Geometry check sheet. Reference: the model listing, model coordinates, mm. Face numbers are marked on the shaded views. Coordinates: 2 decimals unless noted, no trailing zeros. Order: outer loops, then holes, each group sorted by start corner. A loop starts at its lowest first (then second) coordinate and runs counter-clockwise, first axis right, second up. Notation, with made-up numbers: (-22.75, -8.5) - (-1.75, -8.5) arc R12 cw to (-1.75, -0.5) - close; hole circle Ø3 at (58, 37.5). An arc over 180 degrees is marked (long way). Use CSV: the item, a comma, the result in double quotes. Start each with the question number.
1) Draft check along X on the marked faces 1, 2, 3 and 4. Enter one of: released by +X, released by -X, zero draft, split by the parting line, or undercut.
2) Sectioned sample at C-C, the plane z = 6.75. Record the cut outline in (x, y).
3) Thickness scan on probe 1 along Y at (x, z) = (0, 8); probe 2 along X at (y, z) = (-10, 1.25); probe 3 along Y at (x, z) = (2.5, 4). Record the ranges inside material, lowest first. Write a range as [from, to].
4) Sectioned sample at A-A, the plane x = 0. Record the cut outline in (y, z).
5) Sectioned sample at D-D, the plane y = 11. Record the cut outline in (x, z), and give its area (3 significant figures).
6) Depth check by flat-ended pin: P1, Ø21, axis at x = 0, y = 0, coming from the +Z side; P2, Ø2, axis at x = 13, z = 5, coming from the +Y side; P3, Ø1, axis at y = 16, z = 1.5, coming from the +X side. Enter the tip coordinate at first touch or a pass-through.
7) Sectioned sample at B-B, the plane y = -14. Record the cut outline in (x, z).
from build123d import *

# Parameters (mm, degrees)
F1_DEPTH = 10.5


with BuildPart() as f1:
    # F0 (on Top) → F1 (new body)
    with BuildSketch(Plane.XY):
        with BuildLine():
            ThreePointArc((6.061135, 16.244531), (7.933277, 18.430479), (6.899406, 21.116441))
            Line((6.899406, 21.116441), (-21.116441, 21.116441))
            Line((-21.116441, 21.116441), (-21.116441, -21.116441))
            Line((-21.116441, -21.116441), (21.116441, -21.116441))
            Line((21.116441, -21.116441), (21.116441, 6.573539))
            ThreePointArc((21.116441, 6.573539), (18.485123, 8.558267), (16.1976, 6.18546))
            ThreePointArc((16.1976, 6.18546), (17.050859, 3.144896), (17.338459, 0))
            ThreePointArc((17.338459, 0), (-14.242768, -9.887654), (6.061135, 16.244531))
        make_face()
    extrude(amount=F1_DEPTH)


solid = f1.part
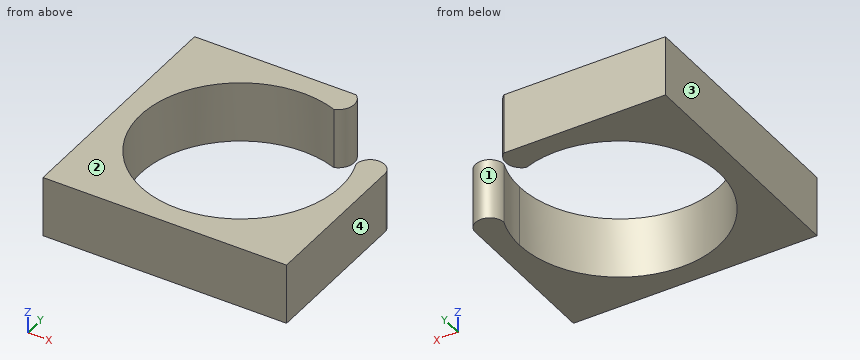
Evaluation:
1,face 1,"undercut"
1,face 2,"zero draft"
1,face 3,"released by -X"
1,face 4,"released by +X"
2,outline,"(-21.12, -21.12) - (21.12, -21.12) - (21.12, 6.57) arc R2.49 ccw to (16.2, 6.19) arc R17.34 cw to (17.34, 0) arc R17.34 cw (long way) to (6.06, 16.24) arc R2.81 ccw to (6.9, 21.12) - (-21.12, 21.12) - close"
3,probe 1,"[-21.12, -17.34], [17.34, 21.12]"
3,probe 2,"[-21.12, -14.16], [14.16, 21.12]"
3,probe 3,"[-21.12, -17.16], [17.16, 21.12]"
4,outline,"(-21.12, 0) - (-17.34, 0) - (-17.34, 10.5) - (-21.12, 10.5) - close; (17.34, 0) - (21.12, 0) - (21.12, 10.5) - (17.34, 10.5) - close"
5,outline,"(-21.12, 0) - (-13.4, 0) - (-13.4, 10.5) - (-21.12, 10.5) - close"
5,area,"81.0 mm²"
6,P1,"through"
6,P2,"y = -10.23"
6,P3,"x = 6.61"
7,outline,"(-21.12, 0) - (-10.23, 0) - (-10.23, 10.5) - (-21.12, 10.5) - close; (10.23, 0) - (21.12, 0) - (21.12, 10.5) - (10.23, 10.5) - close"
